```python
from build123d import *

# Parameters (mm, degrees)
BOSS_EXTRUDE1_DEPTH = 20
FILLET2_R           = 12.7
SKETCH2_R           = 5
SKETCH2_R_2         = 3.75
CUT_EXTRUDE1_DEPTH  = 166.94214143


with BuildPart() as part:
    # Sketch1 → Boss-Extrude1 (new body)
    with BuildSketch(Plane.XY):
        Polygon((10, 0), (10, 25), (50, 48.094010768), (150, 48.094010768), (150, 68.094010768), (50, 68.094010768), (-10, 33.452994616), (-10, 0), align=None)
    extrude(amount=BOSS_EXTRUDE1_DEPTH)

    # Fillet2
    fillet2_edges = [part.edges().sort_by_distance(p)[0] for p in [
        (-10, 33.452994616, 10),
        (50, 68.094010768, 10),
        (50, 48.094010768, 10),
        (10, 25, 10),
    ]]
    fillet(fillet2_edges, radius=FILLET2_R)

    # Sketch2 → Cut-Extrude1 (cut, through all)
    with BuildSketch(Plane.XY.offset(20)):
        with Locations((140, 58.094010768)):
            Circle(SKETCH2_R)
        with Locations((0, 10)):
            Circle(SKETCH2_R_2)
    extrude(amount=-CUT_EXTRUDE1_DEPTH, mode=Mode.SUBTRACT)


solid = part.part
```
The listing builds one solid part. Answer for the finished solid, in the listing's coordinates (mm). A direction names the side the tool comes from. Give positions to 0.01 mm unless a question says otherwise; leave off trailing zeros. Order: outer loops, then holes, each group sorted by start corner. A loop starts at its lowest first (then second) coordinate and runs counter-clockwise, first axis right, second up.
Item 1: The part is cut by section D-D, the plane x = 66.5. Give the vertices of the cut face in (y, z), and give its area (3 significant figures).
From the geometry:
outline: (48.09, 0) - (68.09, 0) - (68.09, 20) - (48.09, 20) - close
area: 400 mm2
Item 2: The part is cut by section C-C, the plane z = 5.5. Give the vertices of the cut face in (x, y), and give its area (3 significant figures).
From the geometry:
outline: (-10, 0) - (10, 0) - (10, 17.67) arc R12.7 cw to (16.35, 28.67) - (47.05, 46.39) arc R12.7 cw to (53.4, 48.09) - (150, 48.09) - (150, 68.09) - (53.4, 68.09) arc R12.7 ccw to (47.05, 66.39) - (-3.65, 37.12) arc R12.7 ccw to (-10, 26.12) - close; hole circle Ø7.5 at (0, 10); hole circle Ø10 at (140, 58.09)
area: 3,460 mm2
Item 3: The part is cut by section B-B, the plane x = 0. Give the vertices of the cut face in (y, z).
From the geometry:
outline: (0, 0) - (6.25, 0) - (6.25, 20) - (0, 20) - close; (13.75, 0) - (39.23, 0) - (39.23, 20) - (13.75, 20) - close
Item 4: Which of the six approach directions +Z, -Z, +X, -X, +Y, -Y give full straight-line access (tool end or side, diameter ignored) to faces 1 (the face through (0, 0, 10)), 2 (the face through (10, 9, 10))?
From the geometry:
face 1: +Z, -Z, +X, -X, -Y
face 2: +Z, -Z, +X, -Y
Item 5: Given pin 1 Ø2 at (x, z) = (98.5, 16) entering from -Y; pin 2 Ø1 at (x, z) = (16.5, 8) entering from -Y; pin 3 Ø5 at (y, z) = (34.5, 16) entering from -X, each flat-ended and moving along its own axis, determine where each tip first touches the part or whether it passes through.
From the geometry:
pin 1: stops at y = 48.09
pin 2: stops at y = 28.46
pin 3: stops at x = -8.56
Item 6: For a pull along X with two mould halves and no side action, classify faces 3 (the face through (11.655, 23.937, 10.14)), 4 (the face through (139.35, 63.05, 10.14)), 5 (the face through (-10, 13, 10)), 6 (the face through (101, 48.094, 10)) as pulls with the +X half, pulls with the -X half, needs draft (parallel to the pull), parting line crosses it, or undercut.
From the geometry:
face 3: pulls with the +X half
face 4: undercut
face 5: pulls with the -X half
face 6: needs draft
Item 7: The part is cut by section A-A, the plane y = 10. Give the vertices of the cut face in (x, z), and give its area (3 significant figures).
From the geometry:
outline: (-10, 0) - (-3.75, 0) - (-3.75, 20) - (-10, 20) - close; (3.75, 0) - (10, 0) - (10, 20) - (3.75, 20) - close
area: 250 mm2
Item 8: Find the intervals of material crossed by probe 1 along Y at (x, z) = (140, 14); probe 2 along Y at (x, z) = (77.5, 11.5); probe 3 along X at (y, z) = (14, 2.5), in increasing order.
From the geometry:
probe 1: y = 48.09 to 53.09, 63.09 to 68.09
probe 2: y = 48.09 to 68.09
probe 3: x = -10 to 10
